from build123d import *

# Parameters (mm, degrees)
EXTRUDE_1_DEPTH     = 114.3
CUT_EXTRUDE_1_DEPTH = 101.854
FILLET_2_R          = 50.8
FILLET_3_R          = 50.8
FILLET_4_R          = 50.8
FILLET_5_R          = 50.8


with BuildPart() as part:
    # 草图1 → 凸台-拉伸1 (new, symmetric)
    with BuildSketch(Plane.XY):
        Polygon((500, 0), (500, 88.9), (655.436388473, 209.252423204), (734.238570332, 209.252423204), (734.238570332, 269.428634805), (608.842711428, 269.428634805), (375.688128719, 88.9), (375.688128719, 0), (0, 0), (0, -600), (500, -600), align=None)
    extrude(amount=EXTRUDE_1_DEPTH, both=True)

    # 草图2 → 切除-拉伸1 (cut, symmetric)
    with BuildSketch(Plane.XY):
        Polygon((12.7, -12.7), (12.7, 37.178760919), (353.872470169, 37.178760919), (353.872470169, 355.973839439), (721.538570332, 346.822359749), (721.538570332, 256.728634805), (721.538570332, 221.952423204), (651.094376347, 221.952423204), (487.3, 95.128516047), (487.3, -587.3), (12.7, -587.3), align=None)
    extrude(amount=CUT_EXTRUDE_1_DEPTH, both=True, mode=Mode.SUBTRACT)

    # 圆角2
    fillet_2_edges = [part.edges().sort_by_distance(p)[0] for p in [
        (487.3, 95.128516047, 0),
    ]]
    fillet(fillet_2_edges, radius=FILLET_2_R)

    # 圆角3
    fillet_3_edges = [part.edges().sort_by_distance(p)[0] for p in [
        (651.094376347, 221.952423204, 0),
    ]]
    fillet(fillet_3_edges, radius=FILLET_3_R)

    # 圆角4
    fillet_4_edges = [part.edges().sort_by_distance(p)[0] for p in [
        (608.842711428, 269.428634805, 108.077),
        (608.842711428, 269.428634805, -108.077),
    ]]
    fillet(fillet_4_edges, radius=FILLET_4_R)

    # 圆角5
    fillet_5_edges = [part.edges().sort_by_distance(p)[0] for p in [
        (375.688128719, 88.9, 108.077),
        (375.688128719, 88.9, -108.077),
    ]]
    fillet(fillet_5_edges, radius=FILLET_5_R)


solid = part.part
Build history of the part. All positions in model axes, mm. A direction names the side the tool comes from. Round coordinates to 2 decimals unless told otherwise and drop trailing zeros. Write each loop counter-clockwise with the first axis right and the second up, starting at its lowest first coordinate (ties: lowest second). Pieces come first, ordered by that corner, then holes. Notation, with made-up numbers: M -9.5,2 L 34.5,2 A35 cw 34.5,35 Z; hole C 8.25,-8.75 d10. An arc over 180 degrees is marked long. Answer as a JSON object with one key per item and string values. Group by question number.
(1) Cut at B-B (x = 284.5). Give the cut face in (y, z), and give its area (3 significant figures).
(2) Drill centre lines: L1, parallel to X at y = -246, z = -89.5; L2, parallel to Z at x = 431.5, y = 40; L3, parallel to Y at x = 150.5, z = 7. Where is each one in solid material? Low to high.
(3) Mould opens along X. For faces 6 (the flat face through (280, -256, -114.3)), 7 (the cylindrical face through (381, 86.6, 108.2)), 8 (the flat face through (293, -248, 101.854)), 9 (the flat face through (576.63, 148.234, 1.6)) say: pulls with the +X half, pulls with the -X half, needs draft (parallel to the pull), parting line crosses it, or undercut.
(4) Cut at A-A (y = -284). Give the cut face in (x, z), and give its area (3 significant figures).
(5) Cut at C-C (z = -62.5). Give the cut face in (x, y).
(6) Flat gauge pins, fed straight in: pin 1 (12 mm diameter, centred on x = 501.5, z = -38.5, fed in from -Y); pin 2 (3.5 mm diameter, centred on y = 17, z = -111, fed in from -X); pin 3 (5 mm diameter, centred on x = 317, z = -62.5, fed in from +Y); pin 4 (16 mm diameter, centred on x = 682.5, z = -47.5, fed in from +Y). Where does each tip first touch, or does it go through?
(7) Which spindle directions (+Z, -Z, +X, -X, +Y, -Y) get a long thin tool onto all of the face, cutting with end or side? Do faces 1 (the flat face through (496.65, 182.56, -107.99)), 2 (the flat face through (12.7, -290, 1)), 3 (the flat face through (573.093, 161.557, 1.426)), 4 (the flat face through (694, 209.252, 2)), 5 (the flat face through (724, 269.429, 9)). Say none if no direction does.
Responses:
{
 "1": {"outline": "M -600,-114.3 L 0,-114.3 L 0,-101.85 L -587.3,-101.85 L -587.3,101.85 L 0,101.85 L 0,114.3 L -600,114.3 Z", "area": "17,500 mm2"},
 "2": {"L1": "x = 0 to 12.7, 487.3 to 500", "L2": "z = -114.3 to -101.85, 101.85 to 114.3", "L3": "y = -600 to -587.3"},
 "3": {"face 6": "needs draft", "face 7": "pulls with the -X half", "face 8": "undercut", "face 9": "pulls with the +X half"},
 "4": {"outline": "M 0,-114.3 L 500,-114.3 L 500,114.3 L 0,114.3 Z; hole M 12.7,-101.85 L 487.3,-101.85 L 487.3,101.85 L 12.7,101.85 Z", "area": "17,600 mm2"},
 "5": {"outline": "M 0,-600 L 500,-600 L 500,88.9 L 655.44,209.25 L 734.24,209.25 L 734.24,269.43 L 721.54,269.43 L 721.54,221.95 L 668.46,221.95 A50.8 ccw 637.36,211.32 L 507,110.38 A50.8 ccw 487.3,70.21 L 487.3,-587.3 L 12.7,-587.3 L 12.7,0 L 0,0 Z"},
 "6": {"pin 1": "stops at y = -600", "pin 2": "stops at x = 375.69", "pin 3": "stops at y = -587.3", "pin 4": "stops at y = 221.95"},
 "7": {"face 1": "+Z, -Z, -X, +Y", "face 2": "+Y", "face 3": "-X, +Y", "face 4": "+Z, -Z, +X, -Y", "face 5": "+Z, -Z, +X, -X, +Y"}
}
